For this review, take the finished solid that the model builds, in its own axes (mm). Face numbers are marked on the shaded views. A direction names the side the tool comes from. Coordinates: 2 decimals unless noted, no trailing zeros. Order: outer loops, then holes, each group sorted by start corner. A loop starts at its lowest first (then second) coordinate and runs counter-clockwise, first axis right, second up. Notation, with made-up numbers: (-25.75, 60) -> (4.25, 60) arc R19 ccw to (4.25, 73) -> close; hole circle Ø8 at (15.25, 41). An arc over 180 degrees is marked (long way). Write item = value, one per line. Start each with the question number.
1) Consider section A-A on y = 12. Give the boundary of the cut face in (x, z).
2) Consider section B-B on x = 4. Give the boundary of the cut face in (y, z).
3) Consider section D-D on z = -25. Give the boundary of the cut face in (x, y).
4) Wall thickness on probe 1 along Z at (x, y) = (0, 18.5); probe 2 along Y at (x, z) = (-3.25, -15); probe 3 along Z at (x, y) = (-1.25, -37.5): over which ranges is each line inside the solid? List them lowest first. Write a range as [from, to].
5) Insertion check: pin 1 Ø7.5 at (x, y) = (0.5, -35.5) entering from -Z; pin 2 Ø6 at (x, z) = (-1.5, 12) entering from +Y; pin 3 Ø8 at (x, z) = (-4.5, 14.5) entering from -Y. Each pin has a flat end and moves straight along its axis. Give the tip position at first contact, or say it passes through.
6) Draft analysis for pull direction Z (two halves, no side actions). For the marked faces 4, 5 and 6, state which applies: +Z half, -Z half, draft (parallel to the pull), parting line (faces both ways), or undercut.
7) Machinability: for the marked faces 1, 2 and 3, which of the approach directions +Z, -Z, +X, -X, +Y, -Y give a long, thin tool a straight path to every point of the face, cutting with its end or side? Answer none if there is none.
8) Consider section C-C on y = -39. Give the boundary of the cut face in (x, z).
Autodesk Inventor part; units mm, degrees
ref_plane "YZ Plane" through (0, 0, 0) normal (1, 0, 0) x (0, 1, 0)
ref_plane "XZ Plane" through (0, 0, 0) normal (0, 1, 0) x (-1, 0, 0)
ref_plane "XY Plane" through (0, 0, 0) normal (0, 0, 1) x (1, 0, 0)
sketch "Sketch1" plane through (0, 0, 0) normal (0, 1, 0) x (-1, 0, 0)
  line L0 (-7.5, -30) -> (7.5, -30)
  line L1 (7.5, -30) -> (7.5, 30)
  line L2 (7.5, 30) -> (-7.5, 30)
  line L3 (-7.5, 30) -> (-7.5, -30)
  line L4 (-7.5, -30) -> (7.5, 30) construction
  line L5 (7.5, -30) -> (-7.5, 30) construction
  point P0 (0, 0)
  dimension "d0" = 15
  dimension "d1" = 60
extrude "Extrusion1" add sketch "Sketch1" along normal blind 3
sketch "Sketch2" plane through (0, 3, 0) normal (0, 1, 0) x (1, 0, 0)
  line L0 (-7.5, 30) -> (-7.5, -30)
  line L1 (7.5, 20.5) -> (-7.5, 20.5)
  line L2 (-7.5, 20.5) -> (-7.5, -20.5)
  line L3 (-7.5, -20.5) -> (7.5, -20.5)
  line L4 (7.5, -20.5) -> (7.5, 20.5)
  line L5 (7.5, 20.5) -> (-7.5, -20.5) construction
  line L6 (-7.5, 20.5) -> (7.5, -20.5) construction
  line L7 (7.5, -20.5) -> (-7.5, -20.5)
  line L8 (-7.5, -20.5) -> (-7.5, -30)
  line L9 (-7.5, -30) -> (7.5, -30)
  line L10 (7.5, -30) -> (7.5, -20.5)
  line L11 (7.5, 30) -> (-7.5, 30)
  line L12 (7.5, 20.5) -> (-7.5, 20.5)
  line L13 (-7.5, 20.5) -> (-7.5, 30)
  line L14 (-7.5, 30) -> (7.5, 30)
  line L15 (7.5, 30) -> (7.5, 20.5)
  point P0 (0, 0)
  dimension "d4" = 41
extrude "Extrusion2" add sketch "Sketch2" along normal blind 19 contours L11 L15 L1 L0 | L3 L10 L9 L0
sketch "Sketch3" plane through (-7.5, 0, -30) normal (-1, 0, 0) x (0, 0, 1)
  line L0 (60, 0) -> (0, 0)
  line L1 (60, 0) -> (50, 0)
  line L2 (50, 0) -> (50, -48)
  line L3 (50, -48) -> (60, -48)
  line L4 (60, -48) -> (60, 0)
  point P0 (30, 0)
  dimension "d7" = 10
  dimension "d8" = 48
extrude "Extrusion3" add sketch "Sketch3" against normal blind 15
sketch "Sketch5" plane through (-7.5, 0, -30) normal (-1, 0, 0) x (0, 0, 1)
  line L0 (0, 0) -> (50, 0)
  line L1 (28.3595, 0) -> (50, -21.6405)
  line L2 (50, -48) -> (50, 0)
  line L3 (28.3595, 0) -> (58.9638, 0) construction
  line L4 (50, -21.6405) -> (50, 0)
  line L5 (50, 0) -> (28.3595, 0)
  point P0 (30, 0)
  dimension "d15" = 45
extrude "Extrusion5" add sketch "Sketch5" against normal blind 15
properties part number "ServoSupport" material "PC/ABS Plastic"
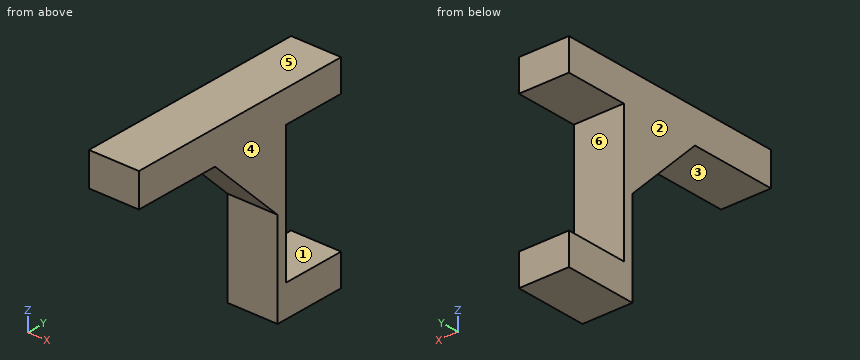
Answer sheet:
q1.outline = (-7.5, -30) -> (7.5, -30) -> (7.5, -20.5) -> (-7.5, -20.5) -> close; (-7.5, 20.5) -> (7.5, 20.5) -> (7.5, 30) -> (-7.5, 30) -> close
q2.outline = (-48, 20) -> (-21.64, 20) -> (0, -1.64) -> (0, -30) -> (22, -30) -> (22, -20.5) -> (3, -20.5) -> (3, 20.5) -> (22, 20.5) -> (22, 30) -> (-48, 30) -> close
q3.outline = (-7.5, 0) -> (7.5, 0) -> (7.5, 22) -> (-7.5, 22) -> close
q4.probe_1 = [-30, -20.5], [20.5, 30]
q4.probe_2 = [0, 3]
q4.probe_3 = [20, 30]
q5.pin_1 = 20
q5.pin_2 = 3
q5.pin_3 = -20.14
q6.face_4 = draft
q6.face_5 = +Z half
q6.face_6 = undercut
q7.face_1 = +X, -X, +Y
q7.face_2 = +Z, -Z, -X, +Y, -Y
q7.face_3 = -Z, +X, -X, -Y
q8.outline = (-7.5, 20) -> (7.5, 20) -> (7.5, 30) -> (-7.5, 30) -> close
